Input: dimensioned drawing with shaded views. Units: mm. Origin: part minimum x, y, z. A direction names the side the tool comes from. Give positions to 0.01 mm unless a question says otherwise; leave off trailing zeros. Write each loop counter-clockwise with the first axis right and the second up, starting at its lowest first coordinate (ties: lowest second). Pieces come first, ordered by that corner, then holes. Notation, with made-up numbers: M 54.25,-29 L 59.25,-29 A22 ccw 59.25,10 Z; hole C 12.25,68 d8. An arc over 180 degrees is marked long. Answer as a JSON object with one key per item and string values.
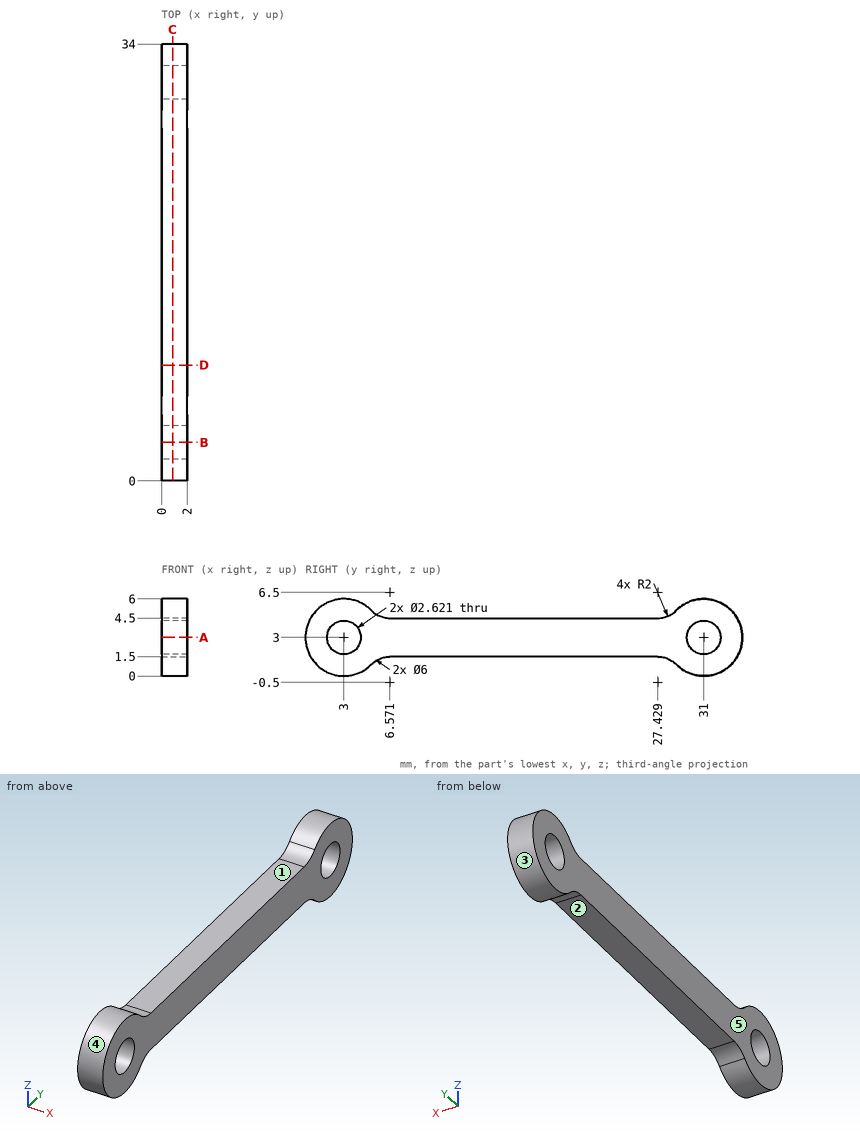
1) Set-up query: the marked faces 1, 2 and 3. Return all of +Z, -Z, +X, -X, +Y, -Y with unobstructed straight access to the full face (end or side cutting, diameter ignored); none if empty.
Geometry check:
{"face 1": "+Z, +X, -X", "face 2": "-Z, +X, -X", "face 3": "+X, -X"}
2) Cut plane A-A on z = 3. Return loops of the section in (x, y).
Geometry check:
{"outline": "M 0,0 L 2,0 L 2,1.69 L 0,1.69 Z; M 0,4.31 L 2,4.31 L 2,29.69 L 0,29.69 Z; M 0,32.31 L 2,32.31 L 2,34 L 0,34 Z"}
3) Pull-direction query (Y, two-part tool) for the marked faces 4 and 5; classes: pulls with the +Y half, pulls with the -Y half, needs draft (parallel to the pull), parting line crosses it, or undercut.
Geometry check:
{"face 4": "undercut", "face 5": "needs draft"}
4) Line query: line 1 (Y direction, x = 0.85, z = 3); line 2 (Y direction, x = 0.25, z = 3.75) (1 decimal); line 3 (Z direction, x = 0.5, y = 31). Output: solid intervals per line, ascending. Write a range as from..to.
Geometry check:
{"line 1": "y = 0..1.69, 4.31..29.69, 32.31..34", "line 2": "y = 0.1..1.9, 4.1..29.9, 32.1..33.9", "line 3": "z = 0..1.69, 4.31..6"}
5) Cut plane C-C on x = 0.85. Return loops of the section in (y, z).
Geometry check:
{"outline": "M 5.14,0.9 A2 cw 6.57,1.5 L 27.43,1.5 A2 cw 28.86,0.9 A3 ccw long 28.86,5.1 A2 cw 27.43,4.5 L 6.57,4.5 A2 cw 5.14,5.1 A3 ccw long Z; hole C 3,3 d2.62; hole C 31,3 d2.62"}
6) Cut plane D-D on y = 9. Return loops of the section in (x, z).
Geometry check:
{"outline": "M 0,1.5 L 2,1.5 L 2,4.5 L 0,4.5 Z"}
7) Cut plane B-B on y = 3. Return loops of the section in (x, z).
Geometry check:
{"outline": "M 0,0 L 2,0 L 2,1.69 L 0,1.69 Z; M 0,4.31 L 2,4.31 L 2,6 L 0,6 Z"}
8) Contact query for flat-ended pins moving along their axis: P1, Ø2.5, axis at y = 3, z = 3, coming from the -X side; P2, Ø1, axis at x = 1, y = 12.5, coming from the +Z side; P3, Ø0.6, axis at x = 1, y = 22, coming from the -Z side. Output: stop coordinate, or through.
Geometry check:
{"P1": "passes through", "P2": "stops at z = 4.5", "P3": "stops at z = 1.5"}
